Design review of the part shown in the three views and the two pictorial views. Dimensions are in mm from the part's minimum x, y and z. A direction names the side the tool comes from. Round coordinates to 2 decimals unless told otherwise and drop trailing zeros. Loops run counter-clockwise (first coordinate to the right, second up) from the corner with the lowest first, then second, coordinate; pieces in that order, holes last. Notation, with made-up numbers: M 6,-26 L 17,-26 A17 ccw 17,5 Z; hole C 25.5,-6 d7. An arc over 180 degrees is marked long. One line per question, with ' | ' between items.
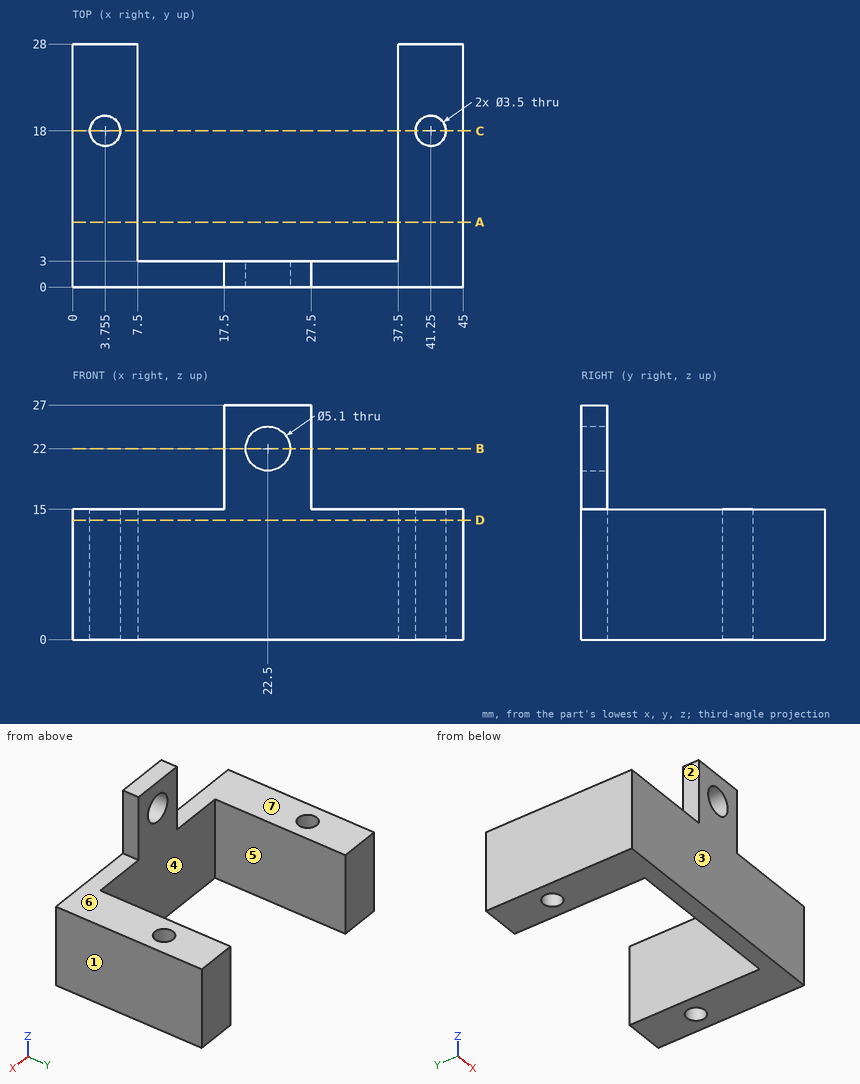
1) Add section B-B on z = 22. State the section outline as (x, y) points, then the cut area to 3 significant figures.
Output values:
outline: M 17.5,0 L 19.95,0 L 19.95,3 L 17.5,3 Z; M 25.05,0 L 27.5,0 L 27.5,3 L 25.05,3 Z | area: 14.7 mm²
2) Add section D-D on z = 13.75. State how many separate pieces and enclosed holes the cut face has, then the cut area to 3 significant figures.
Output values:
separate pieces: 1 | enclosed holes: 2 | area: 491 mm²
3) Insertion check: P1, Ø5, axis at x = 9, y = 7, coming from the +Z side; P2, Ø1.5, axis at y = 1, z = 21.5, coming from the +X side; P3, Ø13.5, axis at x = 17, z = 12, coming from the +Y side; P4, Ø10, axis at x = 39, z = 19.5, coming from the +Y side. Each pin has a flat end and moves straight along its axis. Give the tip position at first contact, or say it passes through.
Output values:
P1: stops at z = 15 | P2: stops at x = 27.5 | P3: stops at y = 3 | P4: stops at y = 28
4) For line 1 (X direction, y = 18, z = 10) (1 decimal); line 2 (Y direction, x = 41.25, z = 6.5); line 3 (X direction, y = 2.05, z = 22), list the stretches that pass through material, from the lowest coordinate up.
Output values:
line 1: x = 0 to 2, 5.5 to 7.5, 37.5 to 39.5, 43 to 45 | line 2: y = 0 to 16.25, 19.75 to 28 | line 3: x = 17.5 to 19.95, 25.05 to 27.5
5) Add section A-A on y = 7.5. State the section outline as (x, z) points.
Output values:
outline: M 0,0 L 7.5,0 L 7.5,15 L 0,15 Z; M 37.5,0 L 45,0 L 45,15 L 37.5,15 Z
6) Add section C-C on y = 18. State the section outline as (x, z) points (1 decimal), then the cut area to 3 significant figures.
Output values:
outline: M 0,0 L 2,0 L 2,15 L 0,15 Z; M 5.5,0 L 7.5,0 L 7.5,15 L 5.5,15 Z; M 37.5,0 L 39.5,0 L 39.5,15 L 37.5,15 Z; M 43,0 L 45,0 L 45,15 L 43,15 Z | area: 120 mm²
7) Mouldability with a two-part tool opening along X and no side actions: class the marked faces 1, 2, 3 and 4 as +X half, -X half, draft (parallel to the pull), parting line (faces both ways), or undercut.
Output values:
face 1: +X half | face 2: -X half | face 3: draft | face 4: undercut
8) Machinability: for the marked faces 5, 6 and 7, which of the approach directions +Z, -Z, +X, -X, +Y, -Y give a long, thin tool a straight path to every point of the face, cutting with its end or side? Answer none if there is none.
Output values:
face 5: +Z, -Z, +Y | face 6: +Z, +X, +Y, -Y | face 7: +Z, -X, +Y, -Y
